Work out the finished part from the listing and answer in its coordinate system (mm). A direction names the side the tool comes from. Round coordinates to 2 decimals unless told otherwise and drop trailing zeros. Loops run counter-clockwise (first coordinate to the right, second up) from the corner with the lowest first, then second, coordinate; pieces in that order, holes last.
```python
from build123d import *

# Parameters (mm, degrees)
F0_W      = 63.5
F0_H      = 127
F1_DEPTH  = 57.658
F2_W      = 50.7999993861
F2_H      = 114.3
F3_DEPTH  = 155.702
F4_W      = 114.3000005424
F4_H      = 44.9580000767
F5_DEPTH  = 96.774
F6_W      = 50.8000007063
F6_H      = 44.9580000767
F7_DEPTH  = 127
F8_DEPTH  = 120.142
F9_DEPTH  = 115.824
F11_DEPTH = 12.7
F13_DEPTH = 25.4
F14_W     = 31.8544553593
F14_H     = 14.1892433167
F15_DEPTH = 5.08
F16_R     = 4.3491356376
F16_R_2   = 3.81
F17_DEPTH = 63.5
F18_DEPTH = 94.488


# Not quite as in the source:
# - after a boolean that leaves OpenCascade's solid faulty, fix() repairs it


with BuildPart() as f1:
    # F0 (on Top) → F1 (new body)
    with BuildSketch(Plane.XY):
        with Locations((4.1889519542, 37.7824994028)):
            Rectangle(F0_W, F0_H)
    extrude(amount=F1_DEPTH)

    # F2 (on face) → F3 (cut)
    with BuildSketch(Plane.XY.offset(57.658)):
        with Locations((4.1889529675, 37.7824994028)):
            Rectangle(F2_W, F2_H)
    extrude(amount=-F3_DEPTH, mode=Mode.SUBTRACT)

    # F4 (on face) → F5 (cut)
    with BuildSketch(Plane.YZ.offset(35.9389519542)):
        with Locations((37.7824991316, 28.8289999616)):
            Rectangle(F4_W, F4_H)
    extrude(amount=-F5_DEPTH, mode=Mode.SUBTRACT)

    # F6 (on face) → F7 (cut)
    with BuildSketch(Plane(origin=(0, 101.2824994028, 0), x_dir=(-1, 0, 0), z_dir=(0, 1, 0))):
        with Locations((-4.1889523074, 28.8289999616)):
            Rectangle(F6_W, F6_H)
    extrude(amount=-F7_DEPTH, mode=Mode.SUBTRACT)

    add(f1.part.fix(), mode=Mode.REPLACE)

    # F8 (add): a face of the model
    f8_faces = [f1.faces().sort_by_distance(p)[0] for p in [
        (4.1889529675, -19.3675005972, 3.1749999616),
    ]]
    extrude(f8_faces, amount=F8_DEPTH)

    # F9 (add): a face of the model
    f9_faces = [f1.faces().sort_by_distance(p)[0] for p in [
        (4.1889529675, -19.3675005972, 54.483),
    ]]
    extrude(f9_faces, amount=F9_DEPTH)

    # F10 (on Top) → F11 (join)
    with BuildSketch(Plane.XY):
        Polygon((4.1889519542, -25.7175005972), (-27.5610480458, -25.7175005972), (4.1889519542, -79.4553607702), align=None)
        Polygon((35.9389519542, -25.7175005972), (4.1889519542, -25.7175005972), (4.1889519542, -79.4553607702), align=None)
    extrude(amount=F11_DEPTH)

    # F12 (on face) → F13 (cut)
    with BuildSketch(Plane.XY.offset(12.7)):
        with BuildLine():
            Line((4.1889519963, -73.0581155537), (4.1889520512, -64.701584864))
            ThreePointArc((4.1889520512, -64.701584864), (-0.0063655555, -68.8798501813), (4.1889519963, -73.0581155537))
        make_face()
        with BuildLine():
            ThreePointArc((4.1889519963, -73.0581155537), (7.1324492077, -71.8283317208), (8.3502344445, -68.8798502088))
            ThreePointArc((8.3502344445, -68.8798502088), (7.1324492271, -65.9313687162), (4.1889520512, -64.701584864))
            Line((4.1889520512, -64.701584864), (4.1889519963, -73.0581155537))
        make_face()
    extrude(amount=-F13_DEPTH, mode=Mode.SUBTRACT)

    # F14 (on face) → F15 (join)
    with BuildSketch(Plane.XY.offset(12.7)):
        with Locations((4.1026878171, -37.0831862092)):
            Rectangle(F14_W, F14_H)
    extrude(amount=F15_DEPTH)

    # F16 (on face) → F17 (join)
    with BuildSketch(Plane(origin=(-27.5610480458, 0, 0), x_dir=(0, -1, 0), z_dir=(-1, 0, 0))):
        with BuildLine():
            Line((-75.0678375838, 0), (-89.0953838825, 0))
            ThreePointArc((-89.0953838825, 0), (-82.0816107331, -10.598487235), (-75.0678375838, 0))
        make_face()
        with Locations((-82.0816107331, -4.520711489)):
            Circle(F16_R, mode=Mode.SUBTRACT)
        with BuildLine():
            Line((-53.4179941057, 0), (-67.4455404045, 0))
            ThreePointArc((-67.4455404045, 0), (-60.4317672551, -10.598487235), (-53.4179941057, 0))
        make_face()
        with Locations((-60.4317672551, -4.520711489)):
            Circle(F16_R_2, mode=Mode.SUBTRACT)
        with BuildLine():
            Line((10.5258625229, 0), (-3.5016837758, 0))
            ThreePointArc((-3.5016837758, 0), (3.5120893735, -10.598487235), (10.5258625229, 0))
        make_face()
        with Locations((3.5120893735, -4.520711489)):
            Circle(F16_R_2, mode=Mode.SUBTRACT)
        with Locations((-82.0816107331, -4.520711489)):
            Circle(F16_R)
        with Locations((-60.4317672551, -4.520711489)):
            Circle(F16_R_2)
        with Locations((3.5120893735, -4.520711489)):
            Circle(F16_R_2)
    extrude(amount=-F17_DEPTH)

    # F16 (on face) → F18 (cut)
    with BuildSketch(Plane(origin=(-27.5610480458, 0, 0), x_dir=(0, -1, 0), z_dir=(-1, 0, 0))):
        with Locations((-82.0816107331, -4.520711489)):
            Circle(F16_R)
        with Locations((-60.4317672551, -4.520711489)):
            Circle(F16_R_2)
        with Locations((3.5120893735, -4.520711489)):
            Circle(F16_R_2)
    extrude(amount=-F18_DEPTH, mode=Mode.SUBTRACT)


solid = f1.part
```
1. Find section D-D (y = -24). Write down the section's boundary in (x, z).
Answer key:
outline: (-27.56, 0) - (35.94, 0) - (35.94, 57.66) - (-27.56, 57.66) - close; hole (-21.21, 6.35) - (29.59, 6.35) - (29.59, 51.31) - (-21.21, 51.31) - close
2. Find section B-B (y = 20). Write down the section's boundary in (x, z).
Answer key:
outline: (-27.56, 0) - (35.94, 0) - (35.94, 6.35) - (-27.56, 6.35) - close; (-27.56, 51.31) - (35.94, 51.31) - (35.94, 57.66) - (-27.56, 57.66) - close
3. Determine the mould class of faces 6 (the face through (33, -19.368, 29)), 7 (the face through (-21.211, 98, 29)), 8 (the face through (-11.91, -52.21, 6.26)) for opening direction X: +X half, -X half, draft (parallel to the pull), parting line (faces both ways), or undercut.
Answer key:
face 6: draft
face 7: undercut
face 8: -X half
4. Which of the six approach directions +Z, -Z, +X, -X, +Y, -Y give full straight-line access (tool end or side, diameter ignored) to faces 1 (the face through (20.03, -37, 15)), 2 (the face through (-24, -19.368, 29)), 3 (the face through (4, 101.282, 3)), 4 (the face through (-27.561, 33, 6)), 5 (the face through (9, -25.718, 52))?
Answer key:
face 1: +Z, +X, +Y, -Y
face 2: +X, -X
face 3: +Z, -Z, +X, -X, +Y
face 4: +Z, -Z, -X, +Y, -Y
face 5: +Z, +X, -X, -Y
5. Given pin 1 (1.5 mm diameter, centred on x = -2.5, z = 16.5, fed in from -Y); pin 2 (9.5 mm diameter, centred on x = -2.5, y = 97, fed in from -Z); pin 3 (5.5 mm diameter, centred on y = -35.5, z = 15, fed in from -X); pin 4 (8 mm diameter, centred on y = 82.08, z = -4.52, fed in from -X), each flat-ended and moving along its own axis, determine where each tip first touches the part or whether it passes through.
Answer key:
pin 1: stops at y = -44.18
pin 2: stops at z = 0
pin 3: stops at x = -22.67
pin 4: passes through
6. Find section A-A (z = 11). Write down the section's boundary in (x, y).
Answer key:
outline: (-27.56, -25.72) - (4.19, -79.46) - (35.94, -25.72) - (35.94, -19.37) - (29.59, -19.37) - (29.59, -25.72) - (-21.21, -25.72) - (-21.21, -19.37) - (-27.56, -19.37) - close; (-27.56, 94.93) - (-21.21, 94.93) - (-21.21, 101.28) - (-27.56, 101.28) - close; (29.59, 94.93) - (35.94, 94.93) - (35.94, 101.28) - (29.59, 101.28) - close; hole circle Ø8.36 at (4.17, -68.88)
7. Consider probe 1 along Z at (x, y) = (-4.5, -4); probe 2 along Y at (x, z) = (16, -0.5); probe 3 along Z at (x, y) = (-9.5, 17.5). Determine where each line is inside the solid, lowest interval first.
Answer key:
probe 1: z = -10.58 to -8.3, -0.74 to 6.35, 51.31 to 57.66
probe 2: y = -10.72 to 3.69, 53.23 to 67.64, 74.88 to 80.42, 83.74 to 89.29
probe 3: z = 0 to 6.35, 51.31 to 57.66
8. Find section C-C (x = 17.5). Write down the section's boundary in (y, z), then the cut area to 3 significant figures.
Answer key:
outline: (-56.93, 0) - (-10.53, 0) arc R7.62 ccw (long way) to (3.5, 0) - (53.42, 0) arc R7.62 ccw (long way) to (67.45, 0) - (75.07, 0) arc R7.62 ccw (long way) to (89.1, 0) - (101.28, 0) - (101.28, 6.35) - (-25.72, 6.35) - (-25.72, 12.7) - (-29.99, 12.7) - (-29.99, 17.78) - (-44.18, 17.78) - (-44.18, 12.7) - (-56.93, 12.7) - close; (-25.72, 51.31) - (101.28, 51.31) - (101.28, 57.66) - (-25.72, 57.66) - close; hole circle Ø7.62 at (-3.51, -4.52); hole circle Ø7.62 at (60.43, -4.52); hole circle Ø8.7 at (82.08, -4.52)
area: 2,340 mm2
